Here's the drawing with two shaded views (mm, measured from the low corner). I have some questions. A direction names the side the tool comes from. Round coordinates to 2 decimals unless told otherwise and drop trailing zeros. Order: outer loops, then holes, each group sorted by start corner. A loop starts at its lowest first (then second) coordinate and runs counter-clockwise, first axis right, second up. Notation, with made-up numbers: (-36.75, 72) - (16.25, 72) arc R23 cw to (16.25, 111) - close; hole circle Ø9 at (59, 51.5). An arc over 180 degrees is marked (long way). One line per item, written item: value.
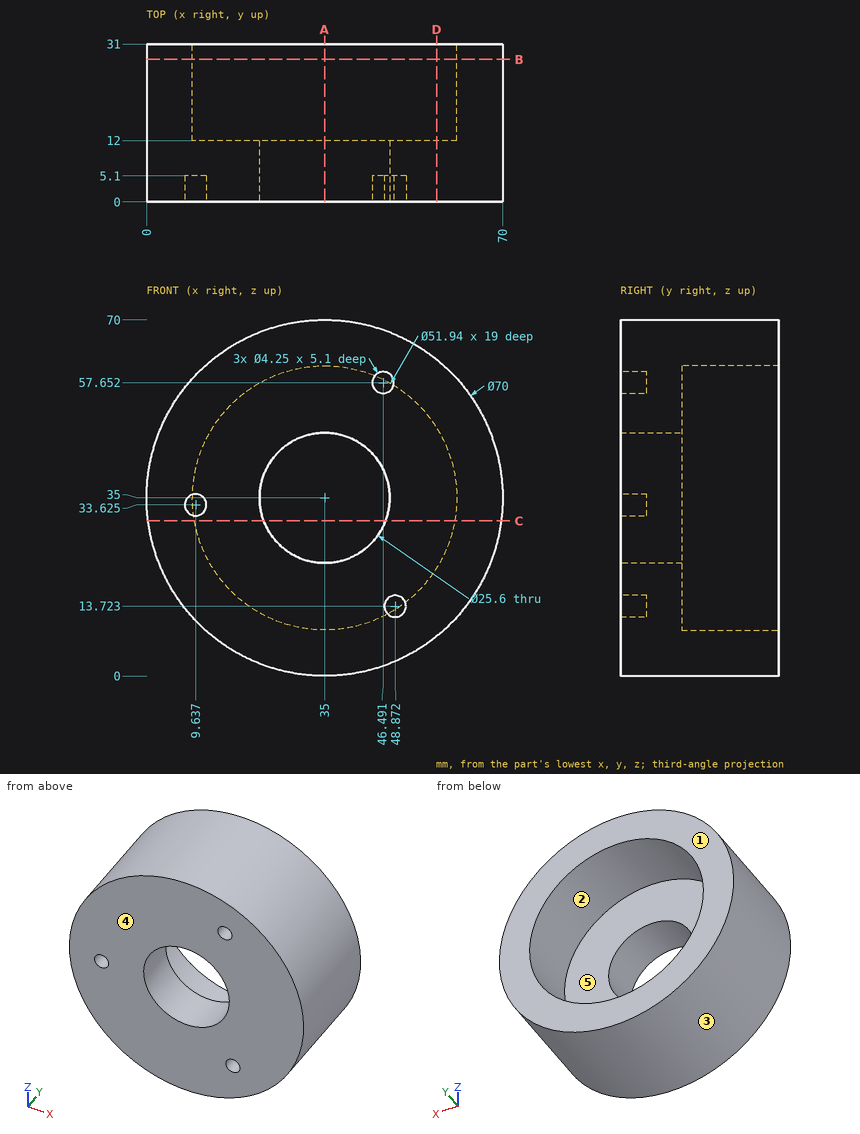
Q1. We'd pull the mould along X, two halves only. Please class the marked faces 3, 4 and 5: released by +X, released by -X, zero draft, split by the parting line, or undercut.
Results list:
face 3: split by the parting line
face 4: zero draft
face 5: undercut
Q2. Which directions (+Z, -Z, +X, -X, +Y, -Y) give clear straight access to the entire face, cutting with the end or side of a thin tool? Please do the marked faces 1 and 2.
Results list:
face 1: +Z, -Z, +X, -X, +Y
face 2: +Y
Q3. Will these pins go through, and if not, where does the flat tip stop? pin 1 (1.3 mm diameter, centred on x = 50, z = 14.5, fed in from -Y); pin 2 (2 mm diameter, centred on y = 25, z = 50.5, fed in from -X) (1 decimal); pin 3 (2 mm diameter, centred on y = 3, z = 9, fed in from -X) (1 decimal).
Results list:
pin 1: y = 5.1
pin 2: x = 3.1
pin 3: x = 10.5
Q4. If we section it at A-A, the plane x = 35: Please give me the cut outline in (y, z).
Results list:
outline: (0, 0) - (31, 0) - (31, 9.03) - (12, 9.03) - (12, 22.2) - (0, 22.2) - close; (0, 47.8) - (12, 47.8) - (12, 60.97) - (31, 60.97) - (31, 70) - (0, 70) - close
Q5. If I drill on line 1 along X through (y, z) = (2.5, 35) (1 decimal); line 2 along X through (y, z) = (14.5, 12) (1 decimal); line 3 along X through (y, z) = (12.5, 36.5), over which ranges is the centre line in solid material (lowest first)?
Results list:
line 1: 0 to 8, 11.3 to 22.2, 47.8 to 70
line 2: 8.6 to 22.9, 47.1 to 61.4
line 3: 0.03 to 9.07, 60.93 to 69.97
Q6. If we section it at B-B, the plane y = 28: Please give me the cut outline in (x, z), then the cut area to 3 significant figures.
Results list:
outline: circle Ø70 at (35, 35); hole circle Ø51.94 at (35, 35)
area: 1,730 mm²
Q7. If we section it at C-C, the plane z = 30.5: Please give me the cut outline in (x, y).
Results list:
outline: (0.29, 0) - (23.02, 0) - (23.02, 12) - (9.42, 12) - (9.42, 31) - (0.29, 31) - close; (46.98, 0) - (69.71, 0) - (69.71, 31) - (60.58, 31) - (60.58, 12) - (46.98, 12) - close
Q8. If we section it at D-D, the plane x = 57: Please give me the cut outline in (y, z).
Results list:
outline: (0, 7.78) - (31, 7.78) - (31, 21.2) - (12, 21.2) - (12, 48.8) - (31, 48.8) - (31, 62.22) - (0, 62.22) - close
